Check sheet for the modelled part. Datum: model origin and axes. Units: mm. Face numbers are marked on the shaded views. A direction names the side the tool comes from. Round coordinates to 2 decimals unless told otherwise and drop trailing zeros. Write each loop counter-clockwise with the first axis right and the second up, starting at its lowest first coordinate (ties: lowest second). Pieces come first, ordered by that corner, then holes. Notation, with made-up numbers: (65.25, 65.25) -> (122.25, 65.25) arc R7 cw to (122.25, 75.25) -> close; hole circle Ø9 at (79.5, 82.25). An arc over 180 degrees is marked (long way). Write item = value, one per line.
from build123d import *

# Parameters (mm, degrees)
BOSS_EXTRUDE1_DEPTH      = 2.5
BOSS_EXTRUDE1_DEPTH_BACK = 2.5
SKETCH1_R                = 78.35
SKETCH1_R_2              = 4
SKETCH1_R_3              = 3
SKETCH1_W                = 100
SKETCH1_H                = 100
BOSS_EXTRUDE2_DEPTH      = 4
BOSS_EXTRUDE2_DEPTH_BACK = 4
SKETCH2_R                = 78.35
SKETCH2_R_2              = 75.35


with BuildPart() as part:
    # Sketch1 → Boss-Extrude1 (new, two sides: drawn at the far end of the back side and taken through both)
    with BuildSketch(Plane(origin=(0, 0, 0), x_dir=(1, 0, 0), z_dir=(0, 1, 0)).offset(-BOSS_EXTRUDE1_DEPTH_BACK)):
        with Locations(Location((0, 0, 0), (0, 0, 270))):
            Circle(SKETCH1_R)
        with Locations(Location((62.5, 0, 0), (0, 0, 270))):
            Circle(SKETCH1_R_2, mode=Mode.SUBTRACT)
        with Locations(Location((-62.5, 0, 0), (0, 0, 270))):
            Circle(SKETCH1_R_2, mode=Mode.SUBTRACT)
        with Locations(Location((0, 62.5, 0), (0, 0, 270))):
            Circle(SKETCH1_R_3, mode=Mode.SUBTRACT)
        with Locations(Location((0, -62.5, 0), (0, 0, 270))):
            Circle(SKETCH1_R_3, mode=Mode.SUBTRACT)
        Rectangle(SKETCH1_W, SKETCH1_H, mode=Mode.SUBTRACT)
    extrude(amount=BOSS_EXTRUDE1_DEPTH + BOSS_EXTRUDE1_DEPTH_BACK)

    # Sketch2 → Boss-Extrude2 (add, two sides: drawn at the far end of the back side and taken through both)
    with BuildSketch(Plane(origin=(0, 0, 0), x_dir=(1, 0, 0), z_dir=(0, 1, 0)).offset(-BOSS_EXTRUDE2_DEPTH_BACK)):
        with Locations(Location((0, 0, 0), (0, 0, 270))):
            Circle(SKETCH2_R)
        with Locations(Location((0, 0, 0), (0, 0, 270))):
            Circle(SKETCH2_R_2, mode=Mode.SUBTRACT)
    extrude(amount=BOSS_EXTRUDE2_DEPTH + BOSS_EXTRUDE2_DEPTH_BACK)


solid = part.part
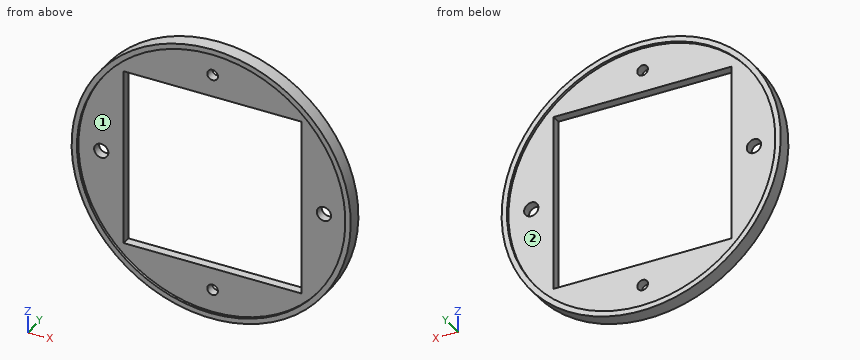
(1) Sectioned sample at C-C on z = -33. Enter the section's corners in (x, y).
Worked answers:
outline = (-71.06, -4) -> (-67.74, -4) -> (-67.74, -2.5) -> (-50, -2.5) -> (-50, 2.5) -> (-67.74, 2.5) -> (-67.74, 4) -> (-71.06, 4) -> close; (50, -2.5) -> (67.74, -2.5) -> (67.74, -4) -> (71.06, -4) -> (71.06, 4) -> (67.74, 4) -> (67.74, 2.5) -> (50, 2.5) -> close
(2) Sectioned sample at B-B on x = 62.5. Enter the section's corners in (y, z), then the cut area to 3 significant figures.
Worked answers:
outline = (-4, -47.25) -> (4, -47.25) -> (4, -42.09) -> (2.5, -42.09) -> (2.5, -4) -> (-2.5, -4) -> (-2.5, -42.09) -> (-4, -42.09) -> close; (-4, 42.09) -> (-2.5, 42.09) -> (-2.5, 4) -> (2.5, 4) -> (2.5, 42.09) -> (4, 42.09) -> (4, 47.25) -> (-4, 47.25) -> close
area = 463 mm²
(3) Access from +Z, -Z, +X, -X, +Y, -Y to the whole of each face (thin tool, end or side, straight path). Record for the marked faces 1 and 2.
Worked answers:
face_1 = -Y
face_2 = +Y
(4) Go/stop test with flat-tipped pins: P1, Ø3.5, axis at x = 0, z = 62.5, coming from the -Y side (3 decimals); P2, Ø5, axis at x = -24, z = -49.5, coming from the +Y side; P3, Ø1.5, axis at x = -48.5, y = -2, coming from the -Z side; P4, Ø7, axis at x = 0, z = -62.5, coming from the -Y side. Record where each tip stops, or that it passes through.
Worked answers:
P1 = through
P2 = 2.5
P3 = -62.12
P4 = -2.5
(5) Sectioned sample at A-A on z = 0. Enter the section's corners in (x, y), then the cut area to 4 significant figures.
Worked answers:
outline = (-78.35, -4) -> (-75.35, -4) -> (-75.35, -2.5) -> (-66.5, -2.5) -> (-66.5, 2.5) -> (-75.35, 2.5) -> (-75.35, 4) -> (-78.35, 4) -> close; (-58.5, -2.5) -> (-50, -2.5) -> (-50, 2.5) -> (-58.5, 2.5) -> close; (50, -2.5) -> (58.5, -2.5) -> (58.5, 2.5) -> (50, 2.5) -> close; (66.5, -2.5) -> (75.35, -2.5) -> (75.35, -4) -> (78.35, -4) -> (78.35, 4) -> (75.35, 4) -> (75.35, 2.5) -> (66.5, 2.5) -> close
area = 221.5 mm²
(6) Sectioned sample at D-D on x = -56.5. Enter the section's corners in (y, z), then the cut area to 3 significant figures.
Worked answers:
outline = (-4, -54.28) -> (4, -54.28) -> (4, -49.85) -> (2.5, -49.85) -> (2.5, 49.85) -> (4, 49.85) -> (4, 54.28) -> (-4, 54.28) -> (-4, 49.85) -> (-2.5, 49.85) -> (-2.5, -49.85) -> (-4, -49.85) -> close
area = 569 mm²
(7) Material ranges on L1, parallel to X at y = 0.1, z = 0; L2, parallel to X at y = -3.1, z = 0; L3, parallel to Z at x = 1, y = 2, recorded low to high. Write a range as [from, to].
Worked answers:
L1 = [-78.35, -66.5], [-58.5, -50], [50, 58.5], [66.5, 78.35]
L2 = [-78.35, -75.35], [75.35, 78.35]
L3 = [-78.34, -65.33], [-59.67, -50], [50, 59.67], [65.33, 78.34]
